Geometry: final body of the model. Coordinates: model frame, mm. A direction names the side the tool comes from. Coordinates: 2 decimals unless noted, no trailing zeros. Order: outer loops, then holes, each group sorted by start corner. A loop starts at its lowest first (then second) coordinate and runs counter-clockwise, first axis right, second up. Notation, with made-up numbers: (87.25, 27.5) -> (136.25, 27.5) arc R29 cw to (136.25, 63.5) -> close; hole circle Ø6 at (-34, -19.5). An arc over 180 degrees is marked (long way). Answer in a Markdown table with one row per item. Add a question column.
1) Section query D-D on y = 3.5. Return the cut outline in (x, z), then the cut area to 3 significant figures.
2) Section query C-C on x = 5.5. Return the cut outline in (y, z).
3) Ray query, line 1 (Z direction, x = 13.5, y = 8.5); line 2 (Y direction, x = 24, z = -7.25); line 3 (Z direction, x = 19, y = 9.25). Return the intervals inside material, ascending. Write a range as from..to.
4) Section query A-A on y = 11. Return the cut outline in (x, z).
5) Pull-direction query (Y, two-part tool) for faces 1 (the face through (7, 10, -3)), 2 (the face through (0, 4, -8)), 3 (the face through (22, 15, -17)); classes: +Y half, -Y half, draft (parallel to the pull), parting line (faces both ways), or undercut.
6) Contact query for flat-ended pins moving along their axis: P1, Ø5.5, axis at y = 6.5, z = -3.5, coming from the +X side; P2, Ø5, axis at x = 14.5, z = -4, coming from the +Y side; P3, Ø4, axis at x = 25.5, y = 18, coming from the +Z side. Output: stop coordinate, or through.
7) Set-up query: faces 4 (the face through (15, 7, -2)), 5 (the face through (22, 10, -17)), 6 (the face through (17, 12, -15)), 7 (the face through (10.07, 12.605, -17.465)). Return all of +Z, -Z, +X, -X, +Y, -Y with unobstructed straight access to the full face (end or side cutting, diameter ignored); none if empty.
8) Section query B-B on z = -18.25. Return the cut outline in (x, y), then the cut area to 3 significant figures.
```python
from build123d import *

# Parameters (mm, degrees)
SKETCH_1_W          = 25
SKETCH_1_H          = 5
SKETCH_1_W_2        = 15
EXTRUDE_1_DEPTH     = 5
SKETCH_1_3_W        = 15
SKETCH_1_3_H        = 5
EXTRUDE_2_DEPTH     = 10
SKETCH_1_4_W        = 25
SKETCH_1_4_H        = 5
EXTRUDE_3_DEPTH     = 20
SKETCH_2_W          = 5
SKETCH_2_H          = 5
CUT_EXTRUDE_1_DEPTH = 20


with BuildPart() as part:
    # Sketch 1 → Extrude 1 (new body)
    with BuildSketch(Plane(origin=(0, 0, 0), x_dir=(1, 0, 0), z_dir=(0, 1, 0))):
        with Locations((17.5, 17.5)):
            Rectangle(SKETCH_1_W, SKETCH_1_H)
        Polygon((15, 0), (20, 0), (30, 10), (30, 15), (5, 15), (5, 20), (0, 20), (0, 5), (15, 5), align=None)
        with Locations((7.5, 2.5)):
            Rectangle(SKETCH_1_W_2, SKETCH_1_H)
    extrude(amount=EXTRUDE_1_DEPTH)

    # Sketch 1_3 → Extrude 2 (add)
    with BuildSketch(Plane(origin=(0, 0, 0), x_dir=(1, 0, 0), z_dir=(0, 1, 0))):
        with Locations((7.5, 2.5)):
            Rectangle(SKETCH_1_3_W, SKETCH_1_3_H)
    extrude(amount=EXTRUDE_2_DEPTH)

    # Sketch 1_4 → Extrude 3 (add)
    with BuildSketch(Plane(origin=(0, 0, 0), x_dir=(1, 0, 0), z_dir=(0, 1, 0))):
        with Locations((17.5, 17.5)):
            Rectangle(SKETCH_1_4_W, SKETCH_1_4_H)
    extrude(amount=EXTRUDE_3_DEPTH)

    # Sketch 2 → Cut-Extrude 1 (cut)
    with BuildSketch(Plane.XY.offset(-15)):
        with Locations((22.5, 12.5)):
            Rectangle(SKETCH_2_W, SKETCH_2_H)
        Polygon((5, 20), (15, 20), (5, 5), align=None)
    extrude(amount=-CUT_EXTRUDE_1_DEPTH, mode=Mode.SUBTRACT)


solid = part.part
```
Result:
| question | item | result |
|---|---|---|
| 1 | outline | (0, -20) -> (30, -20) -> (30, -10) -> (20, 0) -> (0, 0) -> close |
| 1 | area | 550 mm2 |
| 2 | outline | (0, -20) -> (5.75, -20) -> (5.75, -15) -> (5, -15) -> (5, -5) -> (10, -5) -> (10, 0) -> (0, 0) -> close |
| 3 | line 1 | -20..-15, -5..0 |
| 3 | line 2 | 0..5 |
| 3 | line 3 | -20..-15 |
| 4 | outline | (9, -20) -> (20, -20) -> (20, -15) -> (9, -15) -> close; (25, -20) -> (30, -20) -> (30, -15) -> (25, -15) -> close |
| 5 | face 1 | +Y half |
| 5 | face 2 | draft |
| 5 | face 3 | undercut |
| 6 | P1 | x = 25.8 |
| 6 | P2 | y = 10 |
| 6 | P3 | z = -15 |
| 7 | face 4 | +Z, +X, +Y |
| 7 | face 5 | +Z, -Z |
| 7 | face 6 | +X, -X, +Y |
| 7 | face 7 | -Z, -X, +Y |
| 8 | outline | (0, 0) -> (30, 0) -> (30, 20) -> (15, 20) -> (5, 5) -> (0, 5) -> close; hole (20, 10) -> (25, 10) -> (25, 15) -> (20, 15) -> close |
| 8 | area | 425 mm2 |
